For this review, take the finished solid that the model builds, in its own axes (mm). A direction names the side the tool comes from. Round coordinates to 2 decimals unless told otherwise and drop trailing zeros. Write each loop counter-clockwise with the first axis right and the second up, starting at its lowest first coordinate (ties: lowest second). Pieces come first, ordered by that corner, then holes. Notation, with made-up numbers: (74, 53) - (82, 53) arc R26 ccw to (82, 84) - close; hole circle Ø4 at (5, 18.25). An arc over 180 degrees is marked (long way). Answer in a Markdown table with one row per item. Add a question column.
from build123d import *
from build123d.topology import SkipClean

# Parameters (mm, degrees)
SKETCH1_R           = 30
BOSS_EXTRUDE1_DEPTH = 20
SKETCH2_R           = 27.5
CUT_EXTRUDE1_DEPTH  = 47.904157598
BOSS_EXTRUDE2_START = -20
BOSS_EXTRUDE2_DEPTH = 20
SKETCH6_R           = 21.5
CUT_EXTRUDE2_DEPTH  = 35
SKETCH10_R          = 5
CUT_EXTRUDE5_DEPTH  = 120.565881421
SKETCH11_R          = 24
BOSS_EXTRUDE3_DEPTH = 20
BOSS_EXTRUDE4_START = -40
SKETCH12_R          = 24
BOSS_EXTRUDE4_DEPTH = 40
SKETCH13_R          = 21.5
CUT_EXTRUDE6_DEPTH  = 35


with BuildPart() as part:
    # Sketch1 → Boss-Extrude1 (new body)
    with BuildSketch(Plane.XY):
        Circle(SKETCH1_R)
    extrude(amount=BOSS_EXTRUDE1_DEPTH)

    # Sketch2 → Cut-Extrude1 (cut, through all)
    with BuildSketch(Plane.XY.offset(20)):
        Circle(SKETCH2_R)
    extrude(amount=-CUT_EXTRUDE1_DEPTH, mode=Mode.SUBTRACT)

    # Sketch4 → Boss-Extrude2 (add)
    with BuildSketch(Plane.XY.offset(20).offset(BOSS_EXTRUDE2_START)):
        with BuildLine():
            Line((0, 30), (90, 30))
            Line((90, 30), (90, 24))
            ThreePointArc((90, 24), (114, 0), (90, -24))
            Line((90, -24), (90, -30))
            Line((90, -30), (0, -30))
            ThreePointArc((0, -30), (30, 0), (0, 30))
        make_face()
    extrude(amount=BOSS_EXTRUDE2_DEPTH)

    # Sketch6 → Cut-Extrude2 (cut)
    with BuildSketch(Plane.XY.offset(20)):
        with Locations((90, 0)):
            Circle(SKETCH6_R)
    extrude(amount=-CUT_EXTRUDE2_DEPTH, mode=Mode.SUBTRACT)

    # Sketch10 → Cut-Extrude5 (cut, through all)
    with BuildSketch(Plane.XY.offset(20)):
        with Locations((48, 0)):
            Circle(SKETCH10_R)
    extrude(amount=-CUT_EXTRUDE5_DEPTH, mode=Mode.SUBTRACT)

    # Sketch11 → Boss-Extrude3 (add)
    with BuildSketch(Plane.XY.offset(20)):
        with Locations((90, 0)):
            Circle(SKETCH11_R)
    extrude(amount=BOSS_EXTRUDE3_DEPTH)

    # Sketch12 → Boss-Extrude4 (add)
    with SkipClean():  # the faces are left unmerged after this step: merging them gives an invalid solid
        with BuildSketch(Plane.XY.offset(40).offset(BOSS_EXTRUDE4_START)):
            with Locations((90, 0)):
                Circle(SKETCH12_R)
        extrude(amount=BOSS_EXTRUDE4_DEPTH)

    # Sketch13 → Cut-Extrude6 (cut)
    with SkipClean():  # the faces are left unmerged after this step: merging them gives an invalid solid
        with BuildSketch(Plane.XY.offset(40)):
            with Locations((90, 0)):
                Circle(SKETCH13_R)
        extrude(amount=-CUT_EXTRUDE6_DEPTH, mode=Mode.SUBTRACT)


solid = part.part
Q1. Add section D-D on z = 29. State the section outline as (x, y) points, then the cut area to 3 significant figures.
Q2. Draft analysis for pull direction X (two halves, no side actions). For faces 1 (the face through (90, 27, 10)), 2 (the face through (110.507, 6.458, 22.745)), 3 (the face through (44, -6, 20)), state which applies: released by +X, released by -X, zero draft, split by the parting line, or undercut.
Q3. Add section A-A on z = 7.5. State the section outline as (x, y) points, then the cut area to 3 significant figures.
Q4. Insertion check: pin 1 Ø3 at (y, z) = (19.5, 17.5) entering from +X; pin 2 Ø1.8 at (y, z) = (-27.5, 8) entering from +X; pin 3 Ø5 at (x, y) = (57, 12.5) entering from +Z. Each pin has a flat end and moves straight along its axis. Give the tip position at first contact, or say it passes through.
Q5. Add section C-C on y = -11.5. State the section outline as (x, z) points, then the cut area to 3 significant figures.
Q6. To check wall thickness, follow probe 1 along Y at (x, z) = (90, 28.5); probe 2 along Y at (x, z) = (48, 5.5); probe 3 along X at (y, z) = (-10, 19.5). State the ranges of each line that lie inside material, in increasing order.
Q7. Tool access review of faces 4 (the face through (90, -27, 10)), 5 (the face through (90, 0, 5)), 6 (the face through (46, -30, 10)): name each direction out of +Z, -Z, +X, -X, +Y, -Y from which nothing blocks a thin tool from reaching the whole face with its end or side.
Q8. Add section B-B on x = 48. State the section outline as (y, z) points.
Answer sheet:
| question | item | result |
|---|---|---|
| 1 | outline | circle Ø48 at (90, 0); hole circle Ø43 at (90, 0) |
| 1 | area | 357 mm² |
| 2 | face 1 | released by +X |
| 2 | face 2 | undercut |
| 2 | face 3 | zero draft |
| 3 | outline | (0, -30) - (90, -30) - (90, -24) arc R24 ccw to (90, 24) - (90, 30) - (0, 30) arc R30 ccw to start; hole circle Ø55 at (0, 0); hole circle Ø10 at (48, 0); hole circle Ø43 at (90, 0) |
| 3 | area | 3,810 mm² |
| 4 | pin 1 | stops at x = 105.87 |
| 4 | pin 2 | stops at x = 90 |
| 4 | pin 3 | stops at z = 20 |
| 5 | outline | (-27.71, 0) - (-24.98, 0) - (-24.98, 20) - (-27.71, 20) - close; (24.98, 0) - (111.07, 0) - (111.07, 40) - (108.17, 40) - (108.17, 5) - (71.83, 5) - (71.83, 40) - (68.93, 40) - (68.93, 20) - (24.98, 20) - close |
| 5 | area | 1,350 mm² |
| 6 | probe 1 | y = -24 to -21.5, 21.5 to 24 |
| 6 | probe 2 | y = -30 to -5, 5 to 30 |
| 6 | probe 3 | x = -28.28 to -25.62, 25.62 to 70.97, 109.03 to 111.82 |
| 7 | face 4 | +Z, -Z, +X, -Y |
| 7 | face 5 | +Z |
| 7 | face 6 | +Z, -Z, +X, -X, -Y |
| 8 | outline | (-30, 0) - (-5, 0) - (-5, 20) - (-30, 20) - close; (5, 0) - (30, 0) - (30, 20) - (5, 20) - close |
